The model under review builds one solid part; all positions refer to its coordinate system, in mm. Round coordinates to 2 decimals unless told otherwise and drop trailing zeros. Order: outer loops, then holes, each group sorted by start corner. A loop starts at its lowest first (then second) coordinate and runs counter-clockwise, first axis right, second up.
1) Consider section C-C (z = 0.5). Give the number of separate pieces and of enclosed holes in the cut face, then the cut area to 3 significant figures.
2) Clearance check with flat-ended pins moving along their axes: P1, Ø8, axis at x = -65, y = 129.15, coming from the -Z side; P2, Ø5, axis at x = -76.31, y = 140.46, coming from the -Z side; P3, Ø1.2, axis at y = 107, z = -1, coming from the +X side. State where each tip first meets the part, or that it passes through.
3) Consider section B-B (x = -91). Give the boundary of the cut face in (y, z).
4) To check wall thickness, follow L1, parallel to Y at x = -109, z = -0.1; L2, parallel to Y at x = 65, z = 0.45. State the ranges of each line that lie inside material, in increasing order.
5) Mouldability with a two-part tool opening along X and no side actions: class faces 1 (the face through (113.196, 83.139, -0.028)), 2 (the face through (67.999, 134.917, -0.028)), 3 (the face through (-113.196, 83.139, 0.028)), 4 (the face through (-2, 2, -2)) as pulls with the +X half, pulls with the -X half, needs draft (parallel to the pull), parting line crosses it, or undercut.
6) Consider section A-A (x = 65). Give the boundary of the cut face in (y, z).
Autodesk Inventor part; units mm, degrees
ref_plane "YZ Plane" through (0, 0, 0) normal (1, 0, 0) x (0, 1, 0)
ref_plane "XZ Plane" through (0, 0, 0) normal (0, 1, 0) x (-1, 0, 0)
ref_plane "XY Plane" through (0, 0, 0) normal (0, 0, 1) x (1, 0, 0)
sketch "Sketch1" plane through (0, 0, 0) normal (0, 0, 1) x (1, 0, 0)
  line L0 (-115, 145.15) -> (115, 145.15)
  line L1 (115, 145.15) -> (115, -145.15)
  line L2 (115, -145.15) -> (-115, -145.15)
  line L3 (-115, -145.15) -> (-115, 145.15)
  line L4 (-115, 145.15) -> (-85, 145.15)
  line L5 (-85, 145.15) -> (-85, 84.85)
  line L6 (-85, 84.85) -> (-115, 84.85)
  line L7 (-115, 84.85) -> (-115, 145.15)
  line L8 (115, 145.15) -> (85, 145.15)
  line L9 (85, 145.15) -> (85, 84.85)
  line L10 (85, 84.85) -> (115, 84.85)
  line L11 (115, 84.85) -> (115, 145.15)
  circle A0 centre (-65, 129.15) radius 6.5
  circle A1 centre (65, 129.15) radius 6.5
  circle A2 centre (0, 129.15) radius 6
  line L12 (65, 129.15) -> (-65, 129.15) construction
  circle A3 centre (-109, 78.85) radius 3
  circle A4 centre (109, 78.85) radius 3
  circle A5 centre (109, -139.15) radius 3
  circle A6 centre (-109, -139.15) radius 3
  line L13 (109, -139.15) -> (-109, -139.15) construction
  line L14 (109, -139.15) -> (109, 78.85) construction
  line L15 (-109, 78.85) -> (-109, -139.15) construction
  line L16 (109, 78.85) -> (-109, 78.85) construction
  point P0 (0, 0)
  dimension "d0" = 290.3
  dimension "d1" = 230
  dimension "d2" = 30
  dimension "d3" = 30
  dimension "d4" = 60.3
  dimension "d5" = 13
  dimension "d6" = 13
  dimension "d7" = 12
  dimension "d8" = 130
  dimension "d9" = 65
  dimension "d10" = 16
  dimension "d11" = 6
  dimension "d12" = 6
  dimension "d13" = 6
  dimension "d14" = 6
  dimension "d15" = 218
  dimension "d16" = 218
  dimension "d17" = 218
  dimension "d18" = 218
  dimension "d19" = 115
  dimension "d20" = 145.15
  dimension "d21" = 6
  dimension "d22" = 6
extrude "Tykkelse" add sketch "Sketch1" along normal mid plane 4 contours L0 L9 L10 L1 L2 L3 L6 L5
fillet "Fillet1" radius 6 4 edges at (115, -145.15, 0) (-115, -145.15, 0) (-115, 84.85, 0) (115, 84.85, 0)
fillet "Fillet2" radius 3 4 edges at (-85, 84.85, 0) (-85, 145.15, 0) (85, 84.85, 0) (85, 145.15, 0)
sketch "Sketch2" plane through (0, 0, 2) normal (0, 0, 1) x (1, 0, 0)
  line L0 (78, 145.15) -> (81, 142.15)
  line L1 (78, 145.15) -> (52, 145.15)
  line L2 (49, 142.15) -> (52, 145.15)
  line L3 (49, 142.15) -> (49, 116.15)
  line L4 (52, 113.15) -> (49, 116.15)
  line L5 (52, 113.15) -> (78, 113.15)
  line L6 (81, 116.15) -> (78, 113.15)
  line L7 (81, 116.15) -> (81, 142.15)
  circle A0 centre (53.6863, 140.4637) radius 2.25
  circle A1 centre (53.6863, 117.8363) radius 2.25
  circle A2 centre (76.3137, 140.4637) radius 2.25
  circle A3 centre (76.3137, 117.8363) radius 2.25
  circle A4 centre (65, 129.15) radius 10.5
  line L8 (-81, 142.15) -> (-78, 145.15)
  line L9 (-81, 142.15) -> (-81, 116.15)
  line L10 (-78, 113.15) -> (-81, 116.15)
  line L11 (-78, 113.15) -> (-52, 113.15)
  line L12 (-49, 116.15) -> (-52, 113.15)
  line L13 (-49, 116.15) -> (-49, 142.15)
  line L14 (-52, 145.15) -> (-49, 142.15)
  line L15 (-52, 145.15) -> (-78, 145.15)
  circle A5 centre (-76.3137, 117.8363) radius 2.25
  circle A6 centre (-53.6863, 117.8363) radius 2.25
  circle A7 centre (-76.3137, 140.4637) radius 2.25
  circle A8 centre (-53.6863, 140.4637) radius 2.25
  circle A9 centre (-65, 129.15) radius 10.5
  point P0 (0, 0)
extrude "Flange-huller" cut sketch "Sketch2" against normal blind 10 contours A0 | A1 | A2 | A3 | A5 | A6 | A7 | A8
sketch "Sketch3" plane through (0, 0, 2) normal (0, 0, 1) x (1, 0, 0)
  circle A0 centre (0, 129.15) radius 4 construction
  circle A1 centre (0, 121.15) radius 0.75
  circle A2 centre (0, 137.15) radius 0.75
  circle A3 centre (-8, 129.15) radius 0.75
  circle A4 centre (8, 129.15) radius 0.75
  line L0 (0, 137.15) -> (0, 121.15) construction
  line L1 (-8, 129.15) -> (8, 129.15) construction
  circle A5 centre (7.954, 128.2933) radius 0.9464 construction
  circle A6 centre (0, 129.15) radius 8 construction
  point P0 (0, 0)
  dimension "d29" = 1.5
extrude "Flange møtrik" cut sketch "Sketch3" against normal blind 10
equation "\"d3\" = d2"
equation "\"d6\" = d5"
equation "\"d12\" = d11"
equation "\"d13\" = d11"
equation "\"d14\" = d11"
properties part number "Byggeplade Holder mk2"
Answer below:
1. separate pieces: 1
1. enclosed holes: 19
1. area: 62,500 mm2
2. P1: passes through
2. P2: stops at z = -2
2. P3: stops at x = 85
3. outline: (-145.15, -2) - (84.85, -2) - (84.85, 2) - (-145.15, 2) - close
4. L1: y = -145.15 to -142.15, -136.15 to 75.85, 81.85 to 84.85
4. L2: y = -145.15 to 122.65, 135.65 to 145.15
5. face 1: pulls with the +X half
5. face 2: undercut
5. face 3: pulls with the -X half
5. face 4: needs draft
6. outline: (-145.15, -2) - (122.65, -2) - (122.65, 2) - (-145.15, 2) - close; (135.65, -2) - (145.15, -2) - (145.15, 2) - (135.65, 2) - close
